Here's the drawing with two shaded views (mm, measured from the low corner). I have some questions. A direction names the side the tool comes from. Give positions to 0.01 mm unless a question says otherwise; leave off trailing zeros. Loops run counter-clockwise (first coordinate to the right, second up) from the corner with the lowest first, then second, coordinate; pieces in that order, holes last. Notation, with made-up numbers: (2, -17) - (46, -17) arc R31 cw to (46, 14) - close; hole circle Ø2 at (37, 6). An arc over 180 degrees is marked (long way). Answer as a JSON object with one key per item and string values. Group by question number.
Item 1: Please list where these lines run through material, in increasing order: L1, parallel to X at y = 36.5, z = 131.5; L2, parallel to Z at x = 259.5, y = 43.5; L3, parallel to X at y = 32, z = 14.
Item 2: Suppose I cut it at C-C on x = 117.5. Write out the boundary of the cut face in (y, z), and give its area (3 significant figures).
Item 3: Will these pins go through, and if not, where does the flat tip stop? pin 1 (15 mm diameter, centred on y = 37, z = 113, fed in from +X); pin 2 (6 mm diameter, centred on x = 275, z = 43.5, fed in from +Y); pin 3 (9 mm diameter, centred on x = 173.5, y = 36.5, fed in from -Z).
Item 4: Thinking about a two-plate mould opening in X: for the marked faces 4, 5 and 6, which applies, pulls with the +X half, pulls with the -X half, needs draft (parallel to the pull), parting line crosses it, or undercut?
Item 5: Suppose I cut it at B-B on y = 39. Write out the boundary of the cut face in (x, z), and give its area (3 significant figures).
Item 6: Suppose I cut it at A-A on z = 57. Write out the boundary of the cut face in (x, y), and give its area (3 significant figures).
Item 7: Which directions (+Z, -Z, +X, -X, +Y, -Y) give clear straight access to the entire face, cutting with the end or side of a thin tool? Please do the marked faces 1, 2 and 3.
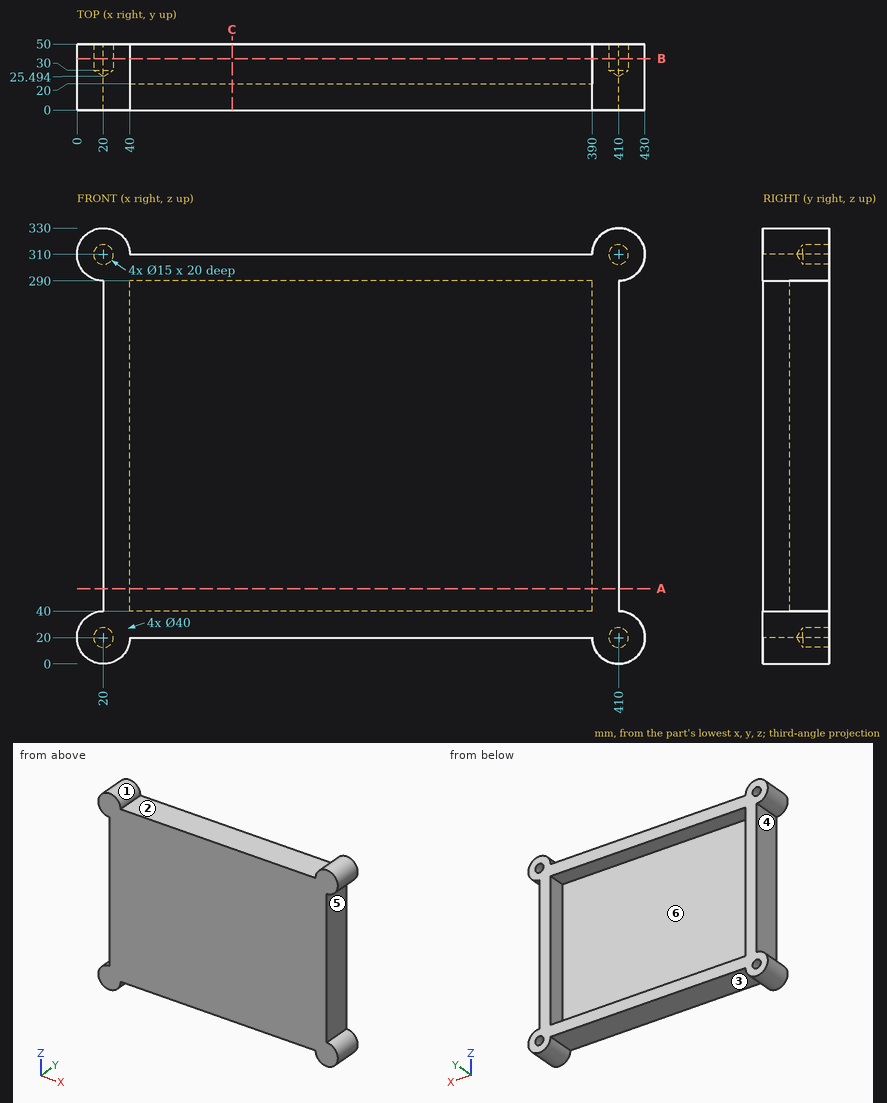
Worked out:
{
 "1": {"L1": "x = 20 to 40, 390 to 410", "L2": "z = 20 to 40, 290 to 310", "L3": "x = 0.92 to 15.5, 24.5 to 39.08, 390.92 to 405.5, 414.5 to 429.08"},
 "2": {"outline": "(0, 20) - (50, 20) - (50, 40) - (20, 40) - (20, 290) - (50, 290) - (50, 310) - (0, 310) - close", "area": "7,000 mm2"},
 "3": {"pin 1": "stops at x = 410", "pin 2": "stops at y = 20", "pin 3": "stops at z = 20"},
 "4": {"face 4": "pulls with the -X half", "face 5": "pulls with the +X half", "face 6": "undercut"},
 "5": {"outline": "(20, 40) arc R20 ccw (long way) to (40, 20) - (390, 20) arc R20 ccw (long way) to (410, 40) - (410, 290) arc R20 ccw (long way) to (390, 310) - (40, 310) arc R20 ccw (long way) to (20, 290) - close; hole circle Ø15 at (20, 20); hole circle Ø15 at (20, 310); hole (40, 40) - (390, 40) - (390, 290) - (40, 290) - close; hole circle Ø15 at (410, 20); hole circle Ø15 at (410, 310)", "area": "28,700 mm2"},
 "6": {"outline": "(20, 0) - (410, 0) - (410, 50) - (390, 50) - (390, 20) - (40, 20) - (40, 50) - (20, 50) - close", "area": "9,000 mm2"},
 "7": {"face 1": "+Y, -Y", "face 2": "+Z, +Y, -Y", "face 3": "-Z, +Y, -Y"}
}
